Verification items for the finished model (mm, model axes). A direction names the side the tool comes from. Coordinates: 2 decimals unless noted, no trailing zeros. Order: outer loops, then holes, each group sorted by start corner. A loop starts at its lowest first (then second) coordinate and runs counter-clockwise, first axis right, second up. Notation, with made-up numbers: M -11.5,45 L 28.5,45 A25 ccw 28.5,80 Z; hole C -27,0 d10. An arc over 180 degrees is marked long. Return JSON: item names as keys, results as strings. Group by question number.
Q1. Thickness scan on probe 1 along X at (y, z) = (0, 1.15); probe 2 along Z at (x, y) = (2.75, -0.5). Record the ranges inside material, lowest first.
Q2. Access from +Z, -Z, +X, -X, +Y, -Y to the whole of each face (thin tool, end or side, straight path). Record for faces 1 (the face through (5.783, 1.574, 6.699)), 2 (the face through (3.58, -2.1, 4.29)).
Q3. Mould release check, pull along X, two halves, no side actions. Record for faces 3 (the face through (-4.42, 4.46, 2.96)), 4 (the face through (4.221, 4.255, 6.699)), 5 (the face through (2, 2, 1.5)): pulls with the +X half, pulls with the -X half, needs draft (parallel to the pull), parting line crosses it, or undercut.
Q4. Section check A-A, the plane z = 5.5. Enter the section's corners in (x, y), then the cut area to 3 significant figures.
Q5. Go/stop test with flat-tipped pins: pin 1 Ø4 at (x, y) = (1.5, -2) entering from +Z; pin 2 Ø5 at (x, y) = (0, 0) entering from +Z. Record where each tip stops, or that it passes through.
from build123d import *

# Parameters (mm, degrees)
PAD_DEPTH       = 7
POCKET_DEPTH    = 5.5
SKETCH002_R     = 2.65
POCKET001_DEPTH = 7.001
FILLET_R        = 1


with BuildPart() as part:
    # Sketch → Pad (new body)
    with BuildSketch(Plane.XY):
        Polygon((5.629165, 3.25), (3.25, 5.629165), (0, 6.5), (-3.25, 5.629165), (-5.629165, 3.25), (-6.5, 0), (-5.629165, -3.25), (-3.25, -5.629165), (0, -6.5), (3.25, -5.629165), (5.629165, -3.25), (6.5, 0), align=None)
    extrude(amount=PAD_DEPTH)

    # Sketch001 (on Face14 of Pad) → Pocket (cut)
    with BuildSketch(Plane.XY.offset(7)):
        Polygon((4.792007, 0), (2.396004, 4.15), (-2.396004, 4.15), (-4.792007, 0), (-2.396004, -4.15), (2.396004, -4.15), align=None)
    extrude(amount=-POCKET_DEPTH, mode=Mode.SUBTRACT)

    # Sketch002 (on DatumPlane) → Pocket001 (cut, through all)
    with BuildSketch(Plane(origin=(0, 0, 0), x_dir=(1, 0, 0), z_dir=(0, 0, -1))):
        Circle(SKETCH002_R)
    extrude(amount=-POCKET001_DEPTH, mode=Mode.SUBTRACT)

    # Fillet
    fillet_edges = [part.edges().sort_by_distance(p)[0] for p in [
        (6.064583, -1.625, 7),
        (6.064583, 1.625, 7),
        (4.439583, 4.439583, 7),
        (1.625, 6.064583, 7),
        (-1.625, 6.064583, 7),
        (-4.439583, 4.439583, 7),
        (-6.064583, 1.625, 7),
        (-6.064583, -1.625, 7),
        (-4.439583, -4.439583, 7),
        (-1.625, -6.064583, 7),
        (1.625, -6.064583, 7),
        (4.439583, -4.439583, 7),
    ]]
    fillet(fillet_edges, radius=FILLET_R)


solid = part.part
Numbers:
{
 "1": {"probe 1": "x = -6.5 to -2.65, 2.65 to 6.5", "probe 2": "z = 0 to 1.5"},
 "2": {"face 1": "+Z, +X, +Y", "face 2": "+Z"},
 "3": {"face 3": "pulls with the -X half", "face 4": "pulls with the +X half", "face 5": "undercut"},
 "4": {"outline": "M -6.5,0 L -5.63,-3.25 L -3.25,-5.63 L 0,-6.5 L 3.25,-5.63 L 5.63,-3.25 L 6.5,0 L 5.63,3.25 L 3.25,5.63 L 0,6.5 L -3.25,5.63 L -5.63,3.25 Z; hole M -4.79,0 L -2.4,-4.15 L 2.4,-4.15 L 4.79,0 L 2.4,4.15 L -2.4,4.15 Z", "area": "67.1 mm2"},
 "5": {"pin 1": "stops at z = 7", "pin 2": "passes through"}
}
